Work out the finished part from the listing and answer in its coordinate system (mm). A direction names the side the tool comes from. Round coordinates to 2 decimals unless told otherwise and drop trailing zeros. Order: outer loops, then holes, each group sorted by start corner. A loop starts at its lowest first (then second) coordinate and runs counter-clockwise, first axis right, second up. Notation, with made-up numbers: M -16,75.25 L 16,75.25 A34 cw 16,110.25 Z; hole C -4.75,44.5 d8. An arc over 180 degrees is marked long. Answer as a JSON object with one key per item and string values. Group by question number.
from build123d import *

# Parameters (mm, degrees)
SKETCH1_R           = 3.175
BOSS_EXTRUDE1_DEPTH = 7.62
BOSS_EXTRUDE2_DEPTH = 5.08
SKETCH4_R           = 1.6383
CUT_EXTRUDE1_DEPTH  = 8.89


with BuildPart() as part:
    # Sketch1 → Boss-Extrude1 (new body)
    with BuildSketch(Plane(origin=(0, 0, 0), x_dir=(1, 0, 0), z_dir=(0, 1, 0))):
        with Locations(Location((0, 0, 0), (0, 0, 90))):
            Circle(SKETCH1_R)
    extrude(amount=BOSS_EXTRUDE1_DEPTH)

    # Sketch3 → Boss-Extrude2 (add)
    with BuildSketch(Plane.XZ):
        Polygon((-1.416669754, 2.841420738), (-3.169077419, 0.193838373), (-1.752407664, -2.647582365), (1.416669754, -2.841420738), (3.169077419, -0.193838373), (1.752407664, 2.647582365), align=None)
    extrude(amount=BOSS_EXTRUDE2_DEPTH)

    # Sketch4 → Cut-Extrude1 (cut)
    with BuildSketch(Plane(origin=(0, 7.62, 0), x_dir=(1, 0, 0), z_dir=(0, 1, 0))):
        with Locations(Location((0, 0, 0), (0, 0, 270))):
            Circle(SKETCH4_R)
    extrude(amount=-CUT_EXTRUDE1_DEPTH, mode=Mode.SUBTRACT)


solid = part.part
Item 1: A tool of negligible diameter and unlimited length cuts with its end or side. For faces 1 (the flat face through (2.42, 0, -1.61)), 2 (the flat face through (-2.47, -2.5, -1.21)), 3 (the flat face through (2.47, -2.5, 1.21)), 4 (the flat face through (-2.28, -2.5, 1.54)), from which of +Z, -Z, +X, -X, +Y, -Y can it reach the whole face along a straight path? Write none if from no direction.
Item 2: Find section B-B (x = -0.25). Give the vertices of the cut face in (y, z), and give its area (3 significant figures).
Item 3: Find section A-A (z = -2.5). Give the vertices of the cut face in (x, y), and give its area (3 significant figures).
Item 4: Consider L1, parallel to X at y = 3.25, z = 0 (3 decimals); L2, parallel to X at y = 0.5, z = -1.75. Determine where each line is inside the solid, lowest interval first.
Item 5: Find section D-D (y = 6.75). Give the vertices of the cut face in (x, z) (3 decimals), and give its area (3 significant figures).
Item 6: The mould has two halves that part along X. Classify faces 5 (the flat face through (0, -1.27, 0)), 6 (the cylindrical face through (1.93, 3.76, 2.52)), 7 (the flat face through (2.6, 0, 1.3)), 8 (the cylindrical face through (1.107, 3.237, -1.207)): +X half, -X half, draft (parallel to the pull), parting line (faces both ways), or undercut.
Item 7: Each of these flat-tipped pins is pushed along its axis until it touches: pin 1 (2.5 mm diameter, centred on x = 0, z = 0, fed in from +Y); pin 2 (0.5 mm diameter, centred on x = 2.5, z = -2, fed in from -Y); pin 3 (1.5 mm diameter, centred on y = -3, z = 2, fed in from +X). Where does it stop, or does it pass through?
Item 8: Find section C-C (y = -3.5). Give the vertices of the cut face in (x, z).
Responses:
{
 "1": {"face 1": "-Z, +X, -Y", "face 2": "-Z, -X, -Y", "face 3": "+Z, +X, -Y", "face 4": "+Z, -X, -Y"},
 "2": {"outline": "M -5.08,-2.74 L 0,-2.74 L 0,-3.17 L 7.62,-3.17 L 7.62,-1.62 L -1.27,-1.62 L -1.27,1.62 L 7.62,1.62 L 7.62,3.17 L 0,3.17 L 0,2.77 L -5.08,2.77 Z", "area": "47.4 mm^2"},
 "3": {"outline": "M -1.96,0 L -1.83,0 L -1.83,-5.08 L 1.64,-5.08 L 1.64,0 L 1.96,0 L 1.96,7.62 L -1.96,7.62 Z", "area": "47.4 mm^2"},
 "4": {"L1": "x = -3.175 to -1.638, 1.638 to 3.175", "L2": "x = -2.65 to 2.65"},
 "5": {"outline": "C 0,0 d6.35; hole C 0,0 d3.277", "area": "23.2 mm^2"},
 "6": {"face 5": "undercut", "face 6": "parting line", "face 7": "draft", "face 8": "undercut"},
 "7": {"pin 1": "stops at y = -1.27", "pin 2": "stops at y = 0", "pin 3": "stops at x = 2.45"},
 "8": {"outline": "M -3.17,0.19 L -1.75,-2.65 L 1.42,-2.84 L 3.17,-0.19 L 1.75,2.65 L -1.42,2.84 Z"}
}
